Part model, mm, in its own coordinate system. A direction names the side the tool comes from. Coordinates: 2 decimals unless noted, no trailing zeros. Write each loop counter-clockwise with the first axis right and the second up, starting at its lowest first coordinate (ties: lowest second). Pieces come first, ordered by that corner, then holes. Notation, with made-up numbers: (31, -8) -> (86, -8) arc R19 ccw to (86, 17) -> close; hole circle Ø11 at (20.5, 62.5). An arc over 180 degrees is marked (long way). Write item = value, one per line.
from build123d import *

# Parameters (mm, degrees)
SKETCH1_W           = 210
SKETCH1_H           = 70
BOSS_EXTRUDE1_DEPTH = 4
SKETCH2_W           = 210
SKETCH2_H           = 4
BOSS_EXTRUDE2_DEPTH = 60
SKETCH3_W           = 4
SKETCH3_H           = 66
BOSS_EXTRUDE3_DEPTH = 30
FILLET1_R           = 10
SKETCH5_W           = 4
SKETCH5_H           = 56
BOSS_EXTRUDE4_DEPTH = 20


with BuildPart() as part:
    # Sketch1 → Boss-Extrude1 (new body)
    with BuildSketch(Plane.XY):
        with Locations((-9.965753425, 84.434931507)):
            Rectangle(SKETCH1_W, SKETCH1_H)
    extrude(amount=BOSS_EXTRUDE1_DEPTH)

    # Sketch2 → Boss-Extrude2 (add)
    with BuildSketch(Plane.XY):
        with Locations((-9.965753425, 51.434931507)):
            Rectangle(SKETCH2_W, SKETCH2_H)
    extrude(amount=-BOSS_EXTRUDE2_DEPTH)

    # Sketch3 → Boss-Extrude3 (add)
    with BuildSketch(Plane.XY):
        with Locations((-112.965753425, 86.434931507)):
            Rectangle(SKETCH3_W, SKETCH3_H)
        with Locations((93.034246575, 86.434931507)):
            Rectangle(SKETCH3_W, SKETCH3_H)
    extrude(amount=-BOSS_EXTRUDE3_DEPTH)

    # Fillet1
    # the kernel refuses this fillet: 10 mm, written as the material it takes off along each edge
    with BuildSketch(Plane(origin=(-110.965753425, 119.434931507, 0), x_dir=(0, 0, 1), z_dir=(1, 0, 0))) as fillet1_piece_1:
        with BuildLine():
            CenterArc((FILLET1_R, FILLET1_R), FILLET1_R, 180, 90)
            Line((0, FILLET1_R), (0, 0))
            Line((0, 0), (FILLET1_R, 0))
        make_face()
    extrude(amount=202, mode=Mode.SUBTRACT)

    # Sketch5 → Boss-Extrude4 (add)
    with BuildSketch(Plane(origin=(0, 0, 0), x_dir=(-1, 0, 0), z_dir=(0, 0, -1))):
        with Locations((9.965753425, 81.434931507)):
            Rectangle(SKETCH5_W, SKETCH5_H)
    extrude(amount=BOSS_EXTRUDE4_DEPTH)


solid = part.part
Q1. Saw through at A-A on z = -6. Give the cut face in (x, y).
Model answer:
outline = (-114.97, 49.43) -> (95.03, 49.43) -> (95.03, 119.43) -> (91.03, 119.43) -> (91.03, 53.43) -> (-7.97, 53.43) -> (-7.97, 109.43) -> (-11.97, 109.43) -> (-11.97, 53.43) -> (-110.97, 53.43) -> (-110.97, 119.43) -> (-114.97, 119.43) -> close
Q2. Saw through at C-C on x = -77. Give the cut face in (y, z), and give its area (3 significant figures).
Model answer:
outline = (49.43, -60) -> (53.43, -60) -> (53.43, 0) -> (109.43, 0) arc R10 ccw to (117.43, 4) -> (49.43, 4) -> close
area = 502 mm²
Q3. Probe line 1 (X direction, y = 96, z = -5); line 2 (X direction, y = 95, z = -25.5); line 3 (Y direction, x = 20, z = -55.5). List the from-to ranges inside material, lowest first. Write a range as from..to.
Model answer:
line_1 = -114.97..-110.97, -11.97..-7.97, 91.03..95.03
line_2 = -114.97..-110.97, 91.03..95.03
line_3 = 49.43..53.43
Q4. Which spindle directions (+Z, -Z, +X, -X, +Y, -Y) get a long thin tool onto all of the face, cutting with end or side? Do faces 1 (the face through (-10, 109.435, -10)), 2 (the face through (93, 119.435, -13)), 3 (the face through (93, 87, -30)). Say none if no direction does.
Model answer:
face_1 = -Z, +Y
face_2 = +Z, -Z, +X, -X, +Y
face_3 = -Z, +X, -X, +Y
Q5. Mould opens along X. For faces 4 (the face through (-114.966, 84, -13)), 5 (the face through (-10, 82, -20)), 6 (the face through (-113, 119.435, -13)), 7 (the face through (91.034, 86, -13)) say: released by +X, released by -X, zero draft, split by the parting line, or undercut.
Model answer:
face_4 = released by -X
face_5 = undercut
face_6 = zero draft
face_7 = undercut
Q6. Saw through at B-B on y = 106. Give the cut face in (x, z), and give its area (3 significant figures).
Model answer:
outline = (-114.97, -30) -> (-110.97, -30) -> (-110.97, 0) -> (-11.97, 0) -> (-11.97, -20) -> (-7.97, -20) -> (-7.97, 0) -> (91.03, 0) -> (91.03, -30) -> (95.03, -30) -> (95.03, 4) -> (-114.97, 4) -> close
area = 1,160 mm²
Q7. Pin check, flat tips, straight feed: pin 1 (4 mm diameter, centred on x = 33, z = -16.5, fed in from +Y); pin 2 (3 mm diameter, centred on x = -10.5, y = 69, fed in from -Z); pin 3 (3 mm diameter, centred on x = 93, y = 89.5, fed in from -Z). Stop position of each tip, or through.
Model answer:
pin_1 = 53.43
pin_2 = -20
pin_3 = -30
Q8. Saw through at D-D on z = -35. Give the cut face in (x, y), and give its area (3 significant figures).
Model answer:
outline = (-114.97, 49.43) -> (95.03, 49.43) -> (95.03, 53.43) -> (-114.97, 53.43) -> close
area = 840 mm²
